Here's the drawing with two shaded views (mm, measured from the low corner). I have some questions. A direction names the side the tool comes from. Coordinates: 2 decimals unless noted, no trailing zeros. Write each loop counter-clockwise with the first axis right and the second up, starting at its lowest first coordinate (ties: lowest second). Pieces come first, ordered by that corner, then holes.
Item 1: I'm going to push flat-ended pins straight in: pin 1 Ø1 at (x, y) = (30.5, 21) entering from +Z; pin 2 Ø10 at (x, y) = (10, 14) entering from -Z; pin 3 Ø10 at (y, z) = (38.5, 28) entering from +X; pin 4 Ø15 at (x, z) = (12.5, 5.5) entering from -Y. Where does each tip first touch, or does it pass through?
Item 2: If we section it at A-A (z = 29.5): Please give me the cut outline in (x, y).
Item 3: If I drill on line 1 (Y direction, x = 13.5, z = 19); line 2 (Z direction, x = 24.5, y = 10.5); line 3 (X direction, y = 31, z = 12), over which ranges is the centre line in solid material (lowest first)?
Item 4: If we section it at B-B (y = 10): Please give me the cut outline in (x, z), then the cut area to 3 significant figures.
Item 5: For the marked faces 1, 2 and 3, which set-ups out of +Z, -Z, +X, -X, +Y, -Y let a thin tool reach every point of the face, with its end or its side?
Item 6: If we section it at C-C (x = 9.5): Please give me the cut outline in (y, z).
Item 7: If we section it at D-D (z = 2): Please give me the cut outline in (x, y), then the cut area to 3 significant figures.
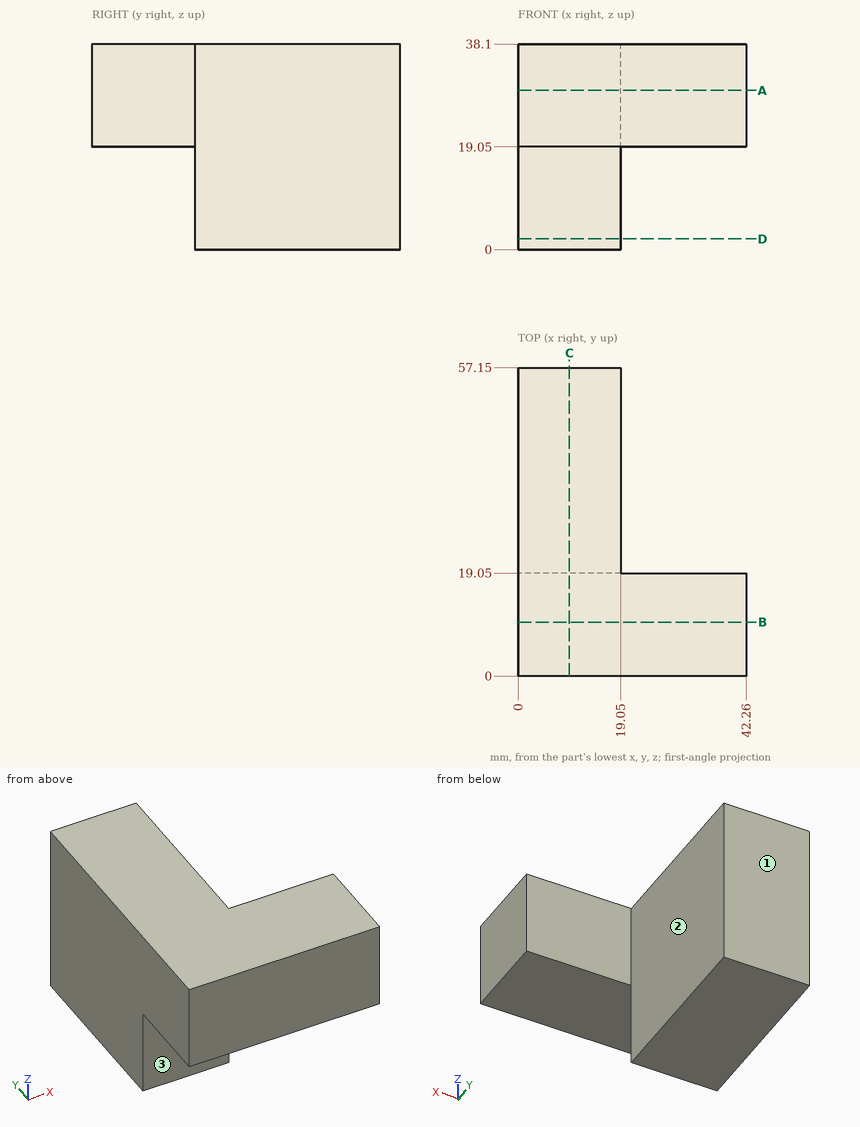
Answer list:
1. pin 1: passes through
1. pin 2: stops at z = 19.05
1. pin 3: stops at x = 19.05
1. pin 4: stops at y = 19.05
2. outline: (0, 0) - (42.26, 0) - (42.26, 19.05) - (19.05, 19.05) - (19.05, 57.15) - (0, 57.15) - close
3. line 1: y = 19.05 to 57.15
3. line 2: z = 19.05 to 38.1
3. line 3: x = 0 to 19.05
4. outline: (0, 19.05) - (42.26, 19.05) - (42.26, 38.1) - (0, 38.1) - close
4. area: 805 mm2
5. face 1: +Z, -Z, +X, -X, +Y
5. face 2: +Z, -Z, +X, +Y
5. face 3: -Z, +X, -X, -Y
6. outline: (0, 19.05) - (19.05, 19.05) - (19.05, 0) - (57.15, 0) - (57.15, 38.1) - (0, 38.1) - close
7. outline: (0, 19.05) - (19.05, 19.05) - (19.05, 57.15) - (0, 57.15) - close
7. area: 726 mm2
